Source: CAD feature listing. Evaluate the final solid. Frame: model axes, mm. Face numbers are marked on the shaded views. A direction names the side the tool comes from. Coordinates: 2 decimals unless noted, no trailing zeros. Order: outer loops, then holes, each group sorted by start corner. A loop starts at its lowest first (then second) coordinate and runs counter-clockwise, first axis right, second up.
```python
from build123d import *

# Parameters (mm, degrees)
SKETCH1_R           = 60
BOSS_EXTRUDE1_DEPTH = 7.5
BOSS_EXTRUDE2_DEPTH = 15
CIRPATTERN1_START   = -7.5
CIRPATTERN1_DEPTH   = 15
SKETCH3_R           = 20
BOSS_EXTRUDE3_DEPTH = 20
CUT_EXTRUDE1_DEPTH  = 103.198336581
CUT_EXTRUDE4_START  = -7.5
SKETCH5_R           = 52.5
SKETCH5_R_2         = 25
CUT_EXTRUDE4_DEPTH  = 3


# Read off the part's stored shape, not the designer's step: CirPattern1
with BuildPart() as part:
    # Sketch1 → Boss-Extrude1 (new, symmetric)
    with BuildSketch(Plane.XY):
        Circle(SKETCH1_R)
    extrude(amount=BOSS_EXTRUDE1_DEPTH, both=True)

    # Sketch2 → Boss-Extrude2 (add)
    with BuildSketch(Plane.XY.offset(7.5)):
        with BuildLine():
            Line((0, 66.5), (0, 60))
            ThreePointArc((0, 60), (2.001113277, 59.966620262), (4, 59.866518188))
            ThreePointArc((4, 59.866518188), (3.099609074, 63.315018359), (1.5, 66.5))
            Line((1.5, 66.5), (0, 66.5))
        make_face()
        with BuildLine():
            ThreePointArc((-4, 59.866518188), (-2.001113277, 59.966620262), (0, 60))
            Line((0, 60), (0, 66.5))
            Line((0, 66.5), (-1.5, 66.5))
            ThreePointArc((-1.5, 66.5), (-3.099609074, 63.315018359), (-4, 59.866518188))
        make_face()
    extrude(amount=-BOSS_EXTRUDE2_DEPTH)

    # CirPattern1 outline → CirPattern1 (add)
    with BuildSketch(Plane.XY.offset(CIRPATTERN1_START)):
        with BuildLine():
            ThreePointArc((-18.660355239, 63.845838881), (-19.381125049, 60.355373564), (-19.358298376, 56.791339868))
            ThreePointArc((-19.358298376, 56.791339868), (-15.529142706, 57.955549577), (-11.630891766, 58.861892228))
            ThreePointArc((-11.630891766, 58.861892228), (-13.393140136, 61.959849286), (-15.76257776, 64.622296016))
            Line((-15.76257776, 64.622296016), (-18.660355239, 63.845838881))
        make_face()
        with BuildLine():
            ThreePointArc((-34.549038106, 56.840689352), (-34.34184938, 53.282609803), (-33.397360709, 49.845925587))
            ThreePointArc((-33.397360709, 49.845925587), (-30, 51.961524227), (-26.469157479, 53.845925587))
            ThreePointArc((-26.469157479, 53.845925587), (-28.973168979, 56.382218877), (-31.950961894, 58.340689352))
            Line((-31.950961894, 58.340689352), (-34.549038106, 56.840689352))
        make_face()
        with BuildLine():
            ThreePointArc((-48.083261121, 45.961940777), (-46.962233428, 42.578724237), (-45.160448102, 39.503593852))
            ThreePointArc((-45.160448102, 39.503593852), (-42.426406871, 42.426406871), (-39.503593852, 45.160448102))
            ThreePointArc((-39.503593852, 45.160448102), (-42.578724237, 46.962233428), (-45.961940777, 48.083261121))
            Line((-45.961940777, 48.083261121), (-48.083261121, 45.961940777))
        make_face()
        with BuildLine():
            ThreePointArc((-58.340689352, 31.950961894), (-56.382218877, 28.973168979), (-53.845925587, 26.469157479))
            ThreePointArc((-53.845925587, 26.469157479), (-51.961524227, 30), (-49.845925587, 33.397360709))
            ThreePointArc((-49.845925587, 33.397360709), (-53.282609803, 34.34184938), (-56.840689352, 34.549038106))
            Line((-56.840689352, 34.549038106), (-58.340689352, 31.950961894))
        make_face()
        with BuildLine():
            ThreePointArc((-64.622296016, 15.76257776), (-61.959849286, 13.393140136), (-58.861892229, 11.630891766))
            ThreePointArc((-58.861892229, 11.630891766), (-57.955549577, 15.529142706), (-56.791339868, 19.358298376))
            ThreePointArc((-56.791339868, 19.358298376), (-60.355373564, 19.381125049), (-63.845838881, 18.660355239))
            Line((-63.845838881, 18.660355239), (-64.622296016, 15.76257776))
        make_face()
        with BuildLine():
            ThreePointArc((-66.5, -1.5), (-63.315018359, -3.099609074), (-59.866518188, -4))
            ThreePointArc((-59.866518188, -4), (-60, 0), (-59.866518188, 4))
            ThreePointArc((-59.866518188, 4), (-63.315018359, 3.099609074), (-66.5, 1.5))
            Line((-66.5, 1.5), (-66.5, -1.5))
        make_face()
        with BuildLine():
            ThreePointArc((-63.845838881, -18.660355239), (-60.355373564, -19.381125049), (-56.791339868, -19.358298376))
            ThreePointArc((-56.791339868, -19.358298376), (-57.955549577, -15.529142706), (-58.861892228, -11.630891766))
            ThreePointArc((-58.861892228, -11.630891766), (-61.959849286, -13.393140136), (-64.622296016, -15.76257776))
            Line((-64.622296016, -15.76257776), (-63.845838881, -18.660355239))
        make_face()
        with BuildLine():
            ThreePointArc((-56.840689352, -34.549038106), (-53.282609803, -34.34184938), (-49.845925587, -33.397360709))
            ThreePointArc((-49.845925587, -33.397360709), (-51.961524227, -30), (-53.845925587, -26.469157479))
            ThreePointArc((-53.845925587, -26.469157479), (-56.382218877, -28.973168979), (-58.340689352, -31.950961894))
            Line((-58.340689352, -31.950961894), (-56.840689352, -34.549038106))
        make_face()
        with BuildLine():
            ThreePointArc((-45.961940777, -48.083261121), (-42.578724237, -46.962233428), (-39.503593852, -45.160448102))
            ThreePointArc((-39.503593852, -45.160448102), (-42.426406871, -42.426406871), (-45.160448102, -39.503593852))
            ThreePointArc((-45.160448102, -39.503593852), (-46.962233428, -42.578724237), (-48.083261121, -45.961940777))
            Line((-48.083261121, -45.961940777), (-45.961940777, -48.083261121))
        make_face()
        with BuildLine():
            ThreePointArc((-31.950961894, -58.340689352), (-28.973168979, -56.382218877), (-26.469157479, -53.845925587))
            ThreePointArc((-26.469157479, -53.845925587), (-30, -51.961524227), (-33.397360709, -49.845925587))
            ThreePointArc((-33.397360709, -49.845925587), (-34.34184938, -53.282609803), (-34.549038106, -56.840689352))
            Line((-34.549038106, -56.840689352), (-31.950961894, -58.340689352))
        make_face()
        with BuildLine():
            ThreePointArc((-15.76257776, -64.622296016), (-13.393140136, -61.959849286), (-11.630891766, -58.861892229))
            ThreePointArc((-11.630891766, -58.861892229), (-15.529142706, -57.955549577), (-19.358298376, -56.791339868))
            ThreePointArc((-19.358298376, -56.791339868), (-19.381125049, -60.355373564), (-18.660355239, -63.845838881))
            Line((-18.660355239, -63.845838881), (-15.76257776, -64.622296016))
        make_face()
        with BuildLine():
            ThreePointArc((1.5, -66.5), (3.099609074, -63.315018359), (4, -59.866518188))
            ThreePointArc((4, -59.866518188), (0, -60), (-4, -59.866518188))
            ThreePointArc((-4, -59.866518188), (-3.099609074, -63.315018359), (-1.5, -66.5))
            Line((-1.5, -66.5), (1.5, -66.5))
        make_face()
        with BuildLine():
            ThreePointArc((18.660355239, -63.845838881), (19.381125049, -60.355373564), (19.358298376, -56.791339868))
            ThreePointArc((19.358298376, -56.791339868), (15.529142706, -57.955549577), (11.630891766, -58.861892229))
            ThreePointArc((11.630891766, -58.861892229), (13.393140136, -61.959849286), (15.76257776, -64.622296016))
            Line((15.76257776, -64.622296016), (18.660355239, -63.845838881))
        make_face()
        with BuildLine():
            ThreePointArc((34.549038106, -56.840689352), (34.34184938, -53.282609803), (33.397360709, -49.845925587))
            ThreePointArc((33.397360709, -49.845925587), (30, -51.961524227), (26.469157479, -53.845925587))
            ThreePointArc((26.469157479, -53.845925587), (28.973168979, -56.382218877), (31.950961894, -58.340689352))
            Line((31.950961894, -58.340689352), (34.549038106, -56.840689352))
        make_face()
        with BuildLine():
            ThreePointArc((48.083261121, -45.961940777), (46.962233428, -42.578724237), (45.160448102, -39.503593852))
            ThreePointArc((45.160448102, -39.503593852), (42.426406871, -42.426406871), (39.503593852, -45.160448102))
            ThreePointArc((39.503593852, -45.160448102), (42.578724237, -46.962233428), (45.961940777, -48.083261121))
            Line((45.961940777, -48.083261121), (48.083261121, -45.961940777))
        make_face()
        with BuildLine():
            ThreePointArc((58.340689352, -31.950961894), (56.382218877, -28.973168979), (53.845925587, -26.469157479))
            ThreePointArc((53.845925587, -26.469157479), (51.961524227, -30), (49.845925587, -33.397360709))
            ThreePointArc((49.845925587, -33.397360709), (53.282609803, -34.34184938), (56.840689352, -34.549038106))
            Line((56.840689352, -34.549038106), (58.340689352, -31.950961894))
        make_face()
        with BuildLine():
            ThreePointArc((64.622296016, -15.76257776), (61.959849286, -13.393140136), (58.861892229, -11.630891766))
            ThreePointArc((58.861892229, -11.630891766), (57.955549577, -15.529142706), (56.791339868, -19.358298376))
            ThreePointArc((56.791339868, -19.358298376), (60.355373564, -19.381125049), (63.845838881, -18.660355239))
            Line((63.845838881, -18.660355239), (64.622296016, -15.76257776))
        make_face()
        with BuildLine():
            ThreePointArc((66.5, 1.5), (63.315018359, 3.099609074), (59.866518188, 4))
            ThreePointArc((59.866518188, 4), (60, 0), (59.866518188, -4))
            ThreePointArc((59.866518188, -4), (63.315018359, -3.099609074), (66.5, -1.5))
            Line((66.5, -1.5), (66.5, 1.5))
        make_face()
        with BuildLine():
            ThreePointArc((63.845838881, 18.660355239), (60.355373564, 19.381125049), (56.791339868, 19.358298376))
            ThreePointArc((56.791339868, 19.358298376), (57.955549577, 15.529142706), (58.861892228, 11.630891766))
            ThreePointArc((58.861892228, 11.630891766), (61.959849286, 13.393140136), (64.622296016, 15.76257776))
            Line((64.622296016, 15.76257776), (63.845838881, 18.660355239))
        make_face()
        with BuildLine():
            ThreePointArc((56.840689352, 34.549038106), (53.282609803, 34.34184938), (49.845925587, 33.397360709))
            ThreePointArc((49.845925587, 33.397360709), (51.961524227, 30), (53.845925587, 26.469157479))
            ThreePointArc((53.845925587, 26.469157479), (56.382218877, 28.973168979), (58.340689352, 31.950961894))
            Line((58.340689352, 31.950961894), (56.840689352, 34.549038106))
        make_face()
        with BuildLine():
            ThreePointArc((45.961940777, 48.083261121), (42.578724237, 46.962233428), (39.503593852, 45.160448102))
            ThreePointArc((39.503593852, 45.160448102), (42.426406871, 42.426406871), (45.160448102, 39.503593852))
            ThreePointArc((45.160448102, 39.503593852), (46.962233428, 42.578724237), (48.083261121, 45.961940777))
            Line((48.083261121, 45.961940777), (45.961940777, 48.083261121))
        make_face()
        with BuildLine():
            ThreePointArc((31.950961894, 58.340689352), (28.973168979, 56.382218877), (26.469157479, 53.845925587))
            ThreePointArc((26.469157479, 53.845925587), (30, 51.961524227), (33.397360709, 49.845925587))
            ThreePointArc((33.397360709, 49.845925587), (34.34184938, 53.282609803), (34.549038106, 56.840689352))
            Line((34.549038106, 56.840689352), (31.950961894, 58.340689352))
        make_face()
        with BuildLine():
            Line((18.660355239, 63.845838881), (15.76257776, 64.622296016))
            ThreePointArc((15.76257776, 64.622296016), (13.393140136, 61.959849286), (11.630891766, 58.861892229))
            ThreePointArc((11.630891766, 58.861892229), (15.529142706, 57.955549577), (19.358298376, 56.791339868))
            ThreePointArc((19.358298376, 56.791339868), (19.381125049, 60.355373564), (18.660355239, 63.845838881))
        make_face()
    extrude(amount=CIRPATTERN1_DEPTH)

    # Sketch3 → Boss-Extrude3 (add, symmetric)
    with BuildSketch(Plane.XY):
        Circle(SKETCH3_R)
    extrude(amount=BOSS_EXTRUDE3_DEPTH, both=True)

    # Sketch4 → Cut-Extrude1 (cut, through all)
    with BuildSketch(Plane(origin=(0, 0, -20), x_dir=(-1, 0, 0), z_dir=(0, 0, -1))):
        with BuildLine():
            Line((-2.5, 9.682458366), (-2.5, 12))
            Line((-2.5, 12), (2.5, 12))
            Line((2.5, 12), (2.5, 9.682458366))
            ThreePointArc((2.5, 9.682458366), (0, -10), (-2.5, 9.682458366))
        make_face()
    extrude(amount=-CUT_EXTRUDE1_DEPTH, mode=Mode.SUBTRACT)

    # Sketch5 → Cut-Extrude4 (cut)
    with BuildSketch(Plane.XY.offset(CUT_EXTRUDE4_START)):
        Circle(SKETCH5_R)
        Circle(SKETCH5_R_2, mode=Mode.SUBTRACT)
    cut_extrude4 = extrude(amount=CUT_EXTRUDE4_DEPTH, mode=Mode.SUBTRACT)

    # Mirror3: Cut-Extrude4 across plane
    add(cut_extrude4.mirror(Plane.XY), mode=Mode.SUBTRACT)


solid = part.part
```
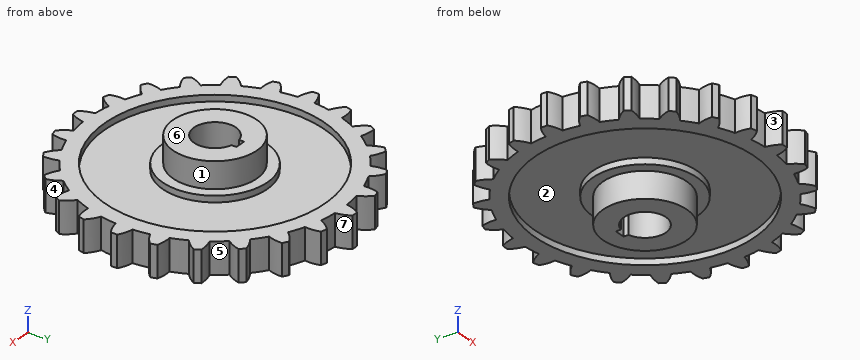
1. Section query B-B, the plane x = -41.5. Output: boundary loops of the cut face in (y, z), plus the area to 3 significant figures.
2. Draft query along Y for the marked faces 5, 6 and 7. Return one class per face: +Y half, -Y half, draft (parallel to the pull), parting line (faces both ways), or undercut.
3. Section query A-A, the plane z = 15.5. Output: boundary loops of the cut face in (x, y).
4. Access query for the marked faces 1, 2, 3 and 4. Directions: +Z, -Z, +X, -X, +Y, -Y. A direction counts if a zero-diameter tool reaches every point of the face in a straight line with its end or side. Return the directions, or none.
5. Contact query for flat-ended pins moving along their axis: P1, Ø5, axis at x = 5, z = 3.5, coming from the +Y side; P2, Ø5, axis at x = -1.5, y = -30, coming from the -Z side; P3, Ø1.5, axis at x = 0, z = 9.5, coming from the -Y side. Output: stop coordinate, or through.
6. Material intervals for line 1 along Y through (x, z) = (0, 5); line 2 along Y through (x, z) = (0, 2); line 3 along Z through (x, y) = (15, -46), sorted ascending.
Answer key:
1. outline: (-46.43, -7.5) - (-32.16, -7.5) - (-32.16, -4.5) - (32.16, -4.5) - (32.16, -7.5) - (46.43, -7.5) - (46.43, 7.5) - (32.16, 7.5) - (32.16, 4.5) - (-32.16, 4.5) - (-32.16, 7.5) - (-46.43, 7.5) - close
1. area: 1,010 mm2
2. face 5: undercut
2. face 6: draft
2. face 7: +Y half
3. outline: circle Ø40 at (0, 0); hole (-2.5, 9.68) arc R10 ccw (long way) to (2.5, 9.68) - (2.5, 12) - (-2.5, 12) - close
4. face 1: +Z
4. face 2: -Z
4. face 3: +Z, -Z, -Y
4. face 4: +Z, -Z, +X
5. P1: stops at y = 64.71
5. P2: stops at z = -4.5
5. P3: stops at y = -20
6. line 1: y = -66.5 to -52.5, -25 to -10, 12 to 25, 52.5 to 66.5
6. line 2: y = -66.5 to -10, 12 to 66.5
6. line 3: z = -4.5 to 4.5
